Part model, mm, in its own coordinate system. Round coordinates to 2 decimals unless told otherwise and drop trailing zeros. Order: outer loops, then holes, each group sorted by start corner. A loop starts at its lowest first (then second) coordinate and runs counter-clockwise, first axis right, second up. Notation, with made-up numbers: (4.25, 38.25) - (15.25, 38.25) arc R18 ccw to (15.25, 65.25) - close; hole circle Ø11 at (60.25, 40.25). An arc over 180 degrees is marked (long way). Answer as a JSON object with one key per item and string values.
```python
from build123d import *


with BuildPart() as part:
    # Szkic1 → Obrót1 (revolve)
    with BuildSketch(Plane.XY):
        with BuildLine():
            Line((0, -46.223602563), (-11.54, -46.223602563))
            Line((-11.54, -46.223602563), (-18.107155743, -45.649050884))
            ThreePointArc((-18.107155743, -45.649050884), (-18.757277337, -45.328446393), (-19.02, -44.652856186))
            Line((-19.02, -44.652856186), (-19.02, 22.516397437))
            ThreePointArc((-19.02, 22.516397437), (-20.191572875, 25.344824562), (-23.02, 26.516397437))
            Line((-23.02, 26.516397437), (-24.42, 26.516397437))
            Line((-24.42, 26.516397437), (-24.425, 26.516397437))
            Line((-24.425, 26.516397437), (-24.425, -54.183602563))
            ThreePointArc((-24.425, -54.183602563), (-24.132106781, -54.890709344), (-23.425, -55.183602563))
            Line((-23.425, -55.183602563), (0, -55.183602563))
            Line((0, -55.183602563), (0, -46.223602563))
        make_face()
    revolve(axis=Axis((0, 49.541128149, 0), (0, -1, 0)))


solid = part.part
```
Item 1: Cut at C-C (y = -22.5). Write the cut outline in (x, z) (3 decimals).
Taken from the geometry:
{"outline": "circle Ø48.85 at (0, 0); hole circle Ø38.04 at (0, 0)"}
Item 2: Cut at B-B (x = 0). Write the cut outline in (y, z) (3 decimals), plus the area to 3 significant figures.
Taken from the geometry:
{"outline": "(-55.184, -23.425) arc R1 ccw to (-54.184, -24.425) - (26.516, -24.425) - (26.516, -23.02) arc R4 ccw to (22.516, -19.02) - (-44.653, -19.02) arc R1 cw to (-45.649, -18.107) - (-46.224, -11.54) - (-46.224, 11.54) - (-45.649, 18.107) arc R1 cw to (-44.653, 19.02) - (22.516, 19.02) arc R4 ccw to (26.516, 23.02) - (26.516, 24.425) - (-54.184, 24.425) arc R1 ccw to (-55.184, 23.425) - close", "area": "1,220 mm2"}
Item 3: Cut at A-A (z = 0). Write the cut outline in (x, y) (3 decimals).
Taken from the geometry:
{"outline": "(-24.425, -54.184) arc R1 ccw to (-23.425, -55.184) - (23.425, -55.184) arc R1 ccw to (24.425, -54.184) - (24.425, 26.516) - (23.02, 26.516) arc R4 ccw to (19.02, 22.516) - (19.02, -44.653) arc R1 cw to (18.107, -45.649) - (11.54, -46.224) - (-11.54, -46.224) - (-18.107, -45.649) arc R1 cw to (-19.02, -44.653) - (-19.02, 22.516) arc R4 ccw to (-23.02, 26.516) - (-24.425, 26.516) - close"}
Item 4: Two-plate mould, pull along Z, no slides. Class faces 1 (the flat face through (0, -55.184, 0)), 2 (the cylindrical face through (-18.142, -10.598, -5.713)), 3 (the cylindrical face through (-23.297, -14.399, -7.337)), 4 (the flat face through (0, -46.224, 0)): pulls with the +Z half, pulls with the -Z half, needs draft (parallel to the pull), parting line crosses it, or undercut.
Taken from the geometry:
{"face 1": "needs draft", "face 2": "undercut", "face 3": "parting line crosses it", "face 4": "undercut"}
Item 5: Probe L1, parallel to X at y = 1, z = 0 (3 decimals); L2, parallel to Y at x = 0.5, z = 5. List the from-to ranges inside material, lowest first. Write a range as from..to.
Taken from the geometry:
{"L1": "-24.425..-19.02, 19.02..24.425", "L2": "-55.18..-46.22"}
Item 6: Drop flat-ended pins along their axis: P1, Ø4, axis at x = -18.5, y = -17.5, coming from the +Z side; P2, Ø8, axis at x = 16.5, y = 2.5, coming from the -Z side; P3, Ø2, axis at x = 15.5, z = 0.5, coming from the +Y side. Give the stop position or say it passes through.
Taken from the geometry:
{"P1": "z = 18.01", "P2": "z = -20.98", "P3": "y = -45.79"}
